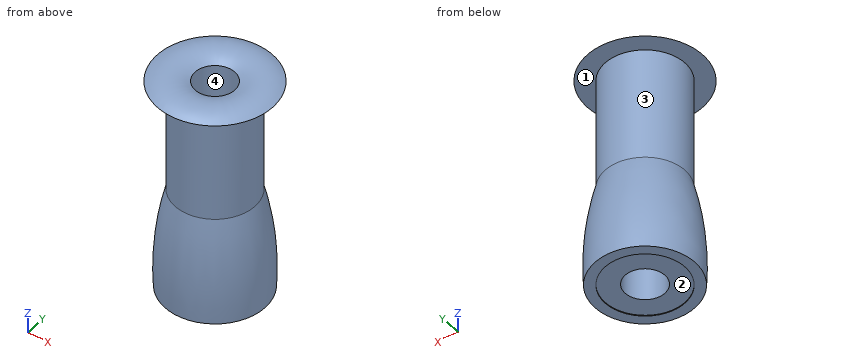
Autodesk Inventor part; units mm, degrees
ref_plane "Work Plane1" through (-20.6161, 18.1675, 0) normal (-1, 0, 0) x (0, 0, 1)
ref_plane "YZ Plane" through (0, 0, 0) normal (1, 0, 0) x (0, 1, 0)
ref_plane "XY Plane" through (0, 0, 0) normal (0, 0, 1) x (1, 0, 0)
sketch "Sketch1" plane through (0, 0, 0) normal (0, 0, 1) x (1, 0, 0)
  circle A0 centre (-20.6161, 18.1675) radius 2.3813
  circle A1 centre (-20.6161, 18.1675) radius 1.1848
  dimension "d0" = 4.7625
extrude "Extrusion1" add sketch "Sketch1" along normal blind 12.7
ref_plane "Work Plane1" through (-20.6161, 18.1675, 0) normal (-1, 0, 0) x (0, 0, 1)
sketch "Sketch2" plane through (-20.6161, 18.1675, 0) normal (-1, 0, 0) x (0, 0, 1)
  line L0 (0, 1.1848) -> (12.7, 1.1848)
  line L1 (0, -1.1848) -> (12.7, -1.1848)
  line L2 (12.7, 1.1848) -> (12.7, -1.1848)
  line L3 (12.7, 2.3813) -> (12.7, -2.3812)
  arc A0 (12.7, 1.1848) -> (12.7, 3.4445) centre (11.0585, 2.3147) ccw
  line L4 (12.7, 3.4445) -> (12.7, 1.1848)
  line L5 (-2.54, 0) -> (15.24, 0)
revolve "Revolution1" add sketch "Sketch2" angle 360 about axis through (-20.6161, 18.1675, 0) along (0, 0, 1)
sketch "Sketch3" plane through (-20.6161, 18.1675, 0) normal (-1, 0, 0) x (0, 0, 1)
  line L0 (12.7, -3.4445) -> (12.7, -2.3812)
  line L1 (12.7, -2.3812) -> (0, -2.3812)
  line L2 (0, -2.3812) -> (0, -1.1848)
  line L3 (0, -1.1848) -> (12.7, -1.1848)
  arc A0 (12.7, -3.4445) -> (12.7, -1.1848) centre (11.0585, -2.3147) ccw
  line L4 (12.7, 2.3813) -> (12.7, 3.4445)
  arc A1 (12.7, 1.1848) -> (12.7, 3.4445) centre (11.0585, 2.3147) ccw
  line L5 (12.7, 1.1848) -> (0, 1.1848)
  line L6 (0, 1.1848) -> (0, 2.3813)
  line L7 (0, 2.3813) -> (12.7, 2.3813)
  line L8 (-2.6102, 0) -> (15.6615, 0)
  arc A2 (5.9963, 2.3813) -> (-0.0511, 2.9836) centre (1.0853, -16.2648) ccw
  line L9 (-0.0511, 2.9836) -> (-0.0511, 2.3813)
  line L10 (5.9963, 2.3813) -> (-0.0511, 2.3813)
  point P0 (6.35, 2.3813)
revolve "Revolution3" add sketch "Sketch3" angle 360 about axis through (-20.6161, 18.1675, 0) along (0, 0, 1) contours L7 L10 L9 A2
properties part number "HW-00010"
The listing builds one solid part. Answer for the finished solid, in the listing's coordinates (mm). Face numbers are marked on the shaded views. Coordinates: 2 decimals unless noted, no trailing zeros. Loops run counter-clockwise (first coordinate to the right, second up) from the corner with the lowest first, then second, coordinate; pieces in that order, holes last. Notation, with made-up numbers: (32, 59) -> (49, 59) arc R28 cw to (49, 93) -> close; hole circle Ø3 at (16, 1.5). An arc over 180 degrees is marked (long way). Answer in a Markdown table with one row per item. Add a question column.
1. Flat-ended cylindrical pins translate along their axes: P1, Ø1.5, axis at x = -19, z = 9.5, coming from the -Y side; P2, Ø3, axis at x = -20.62, y = 18.17, coming from the +Z side; P3, Ø4, axis at y = 19, z = 2, coming from the -X side. Find the tip coordinate at first contact, or state that the pin passes through.
2. Determine the mould class of the marked faces 1, 2, 3 and 4 for opening direction Z: +Z half, -Z half, draft (parallel to the pull), parting line (faces both ways), or undercut.
3. The part is cut by section A-A, the plane z = 11.5. Write down the section's boundary in (x, y).
4. Consider line 1 (X direction, y = 18.25, z = 11.5); line 2 (X direction, y = 19.25, z = 1.75); line 3 (Y direction, x = -20.5, z = 8.25). Determine where each line is inside the solid, lowest interval first. Write a range as [from, to].
Answer below:
| question | item | result |
|---|---|---|
| 1 | P1 | y = 15.95 |
| 1 | P2 | z = 12.88 |
| 1 | P3 | x = -23.63 |
| 2 | face 1 | undercut |
| 2 | face 2 | -Z half |
| 2 | face 3 | undercut |
| 2 | face 4 | draft |
| 3 | outline | circle Ø4.76 at (-20.62, 18.17); hole circle Ø2.37 at (-20.62, 18.17) |
| 4 | line 1 | [-23, -21.8], [-19.43, -18.24] |
| 4 | line 2 | [-23.42, -21.1], [-20.13, -17.81] |
| 4 | line 3 | [15.79, 16.99], [19.35, 20.55] |
